Design review of the part built by this model. Coordinates are the model's own, in mm. A direction names the side the tool comes from. Coordinates: 2 decimals unless noted, no trailing zeros. Loops run counter-clockwise (first coordinate to the right, second up) from the corner with the lowest first, then second, coordinate; pieces in that order, holes last. Notation, with made-up numbers: (-7, -22.5) - (6, -22.5) arc R20 cw to (6, 3.5) - close; hole circle Ø5 at (71.5, 61.5). An arc over 180 degrees is marked (long way). One line per question, with ' | ' between items.
from build123d import *

# Parameters (mm, degrees)
SKETCH1_W           = 12
SKETCH1_H           = 10
BOSS_EXTRUDE1_DEPTH = 9
SKETCH2_R           = 6
BOSS_EXTRUDE2_DEPTH = 15
SKETCH3_R           = 2
BOSS_EXTRUDE3_DEPTH = 1
SKETCH4_R           = 1.25
BOSS_EXTRUDE4_DEPTH = 4.5


with BuildPart() as part:
    # Sketch1 → Boss-Extrude1 (new body)
    with BuildSketch(Plane.XY):
        with Locations((6, -5)):
            Rectangle(SKETCH1_W, SKETCH1_H)
    extrude(amount=BOSS_EXTRUDE1_DEPTH)

    # Sketch2 → Boss-Extrude2 (add)
    with BuildSketch(Plane.XY.offset(9)):
        with Locations((6, -5)):
            Circle(SKETCH2_R)
    extrude(amount=BOSS_EXTRUDE2_DEPTH)

    # Sketch3 → Boss-Extrude3 (add)
    with BuildSketch(Plane(origin=(0, 0, 0), x_dir=(-1, 0, 0), z_dir=(0, 0, -1))):
        with Locations((-6, -5)):
            Circle(SKETCH3_R)
    extrude(amount=BOSS_EXTRUDE3_DEPTH)

    # Sketch4 → Boss-Extrude4 (add)
    with BuildSketch(Plane(origin=(0, 0, -1), x_dir=(-1, 0, 0), z_dir=(0, 0, -1))):
        with Locations((-6, -5)):
            Circle(SKETCH4_R)
    extrude(amount=BOSS_EXTRUDE4_DEPTH)


solid = part.part
Q1. Draft analysis for pull direction X (two halves, no side actions). For faces 5 (the flat face through (12, -5, 4)), 6 (the flat face through (0, -5, 4)), 7 (the flat face through (6, -5, 24)), 8 (the cylindrical face through (0, -5, 16)), state which applies: +X half, -X half, draft (parallel to the pull), parting line (faces both ways), or undercut.
Returned:
face 5: +X half | face 6: -X half | face 7: draft | face 8: parting line
Q2. To check wall thickness, follow line 1 along Z through (x, y) = (8, -4); line 2 along Y through (x, z) = (6.25, 0.25); line 3 along X through (y, z) = (-2.75, 15). State the ranges of each line that lie inside material, in increasing order.
Returned:
line 1: z = 0 to 24 | line 2: y = -10 to 0 | line 3: x = 0.44 to 11.56
Q3. Take a section at C-C (x = 3). Give the boundary of the cut face in (y, z).
Returned:
outline: (-10.2, 9) - (-10, 9) - (-10, 0) - (0, 0) - (0, 9) - (0.2, 9) - (0.2, 24) - (-10.2, 24) - close
Q4. Take a section at A-A (x = 6). Give the boundary of the cut face in (y, z).
Returned:
outline: (-11, 9) - (-10, 9) - (-10, 0) - (-7, 0) - (-7, -1) - (-6.25, -1) - (-6.25, -5.5) - (-3.75, -5.5) - (-3.75, -1) - (-3, -1) - (-3, 0) - (0, 0) - (0, 9) - (1, 9) - (1, 24) - (-11, 24) - close
Q5. Take a section at B-B (y = -9.5). Give the boundary of the cut face in (x, z).
Returned:
outline: (0, 0) - (12, 0) - (12, 9) - (9.97, 9) - (9.97, 24) - (2.03, 24) - (2.03, 9) - (0, 9) - close
Q6. Tool access review of faces 1 (the flat face through (11, -9, 9)), 2 (the flat face through (1, -1, 9)), 3 (the flat face through (5.9, -2.7, 0)), 4 (the flat face through (6, 0, 4)): name each direction out of +Z, -Z, +X, -X, +Y, -Y from which nothing blocks a thin tool from reaching the whole face with its end or side.
Returned:
face 1: +Z, +X, -Y | face 2: +Z, -X, +Y | face 3: -Z | face 4: -Z, +X, -X, +Y
Q7. For pin 1 (1.5 mm diameter, centred on x = 10.5, z = 16, fed in from -Y); pin 2 (4.5 mm diameter, centred on x = 3.5, z = 3.5, fed in from +Y); pin 3 (1.5 mm diameter, centred on y = -1.5, z = 10, fed in from +X), all flat-tipped, find the tip position at first contact; note any pin that passes through.
Returned:
pin 1: stops at y = -9.68 | pin 2: stops at y = 0 | pin 3: stops at x = 11.33
